```python
from build123d import *

# Parameters (mm, degrees)
F0_R     = 177.8
F1_DEPTH = 76.2
F2_R     = 88.9
F3_DEPTH = 254
F4_R     = 69.85
F5_DEPTH = 254
F6_W     = 462.104425
F6_H     = 46.355292
F6_W_2   = 466.450229
F6_H_2   = 34.23076
F7_DEPTH = 254
F8_R     = 158.592368
F9_DEPTH = 12.7


with BuildPart() as f1:
    # F0 (on Top) → F1 (new body)
    with BuildSketch(Plane.XY):
        Circle(F0_R)
    extrude(amount=F1_DEPTH)

    # F2 (on face) → F3 (cut)
    with BuildSketch(Plane.XY.offset(76.2)):
        Circle(F2_R)
    extrude(amount=-F3_DEPTH, mode=Mode.SUBTRACT)

    # F4 (on face) → F5 (cut)
    with BuildSketch(Plane.XY.offset(76.2)):
        with Locations((0, 177.8)):
            Circle(F4_R)
        with Locations((0, -177.8)):
            Circle(F4_R)
    extrude(amount=-F5_DEPTH, mode=Mode.SUBTRACT)

    # F6 (on face) → F7 (cut)
    with BuildSketch(Plane.XY.offset(76.2)):
        with Locations((-1.086809, 155.526124)):
            Rectangle(F6_W, F6_H)
        with Locations((1.086094, -146.964084)):
            Rectangle(F6_W_2, F6_H_2)
    extrude(amount=-F7_DEPTH, mode=Mode.SUBTRACT)

    # F8 (on face) → F9 (cut)
    with BuildSketch(Plane.XY.offset(76.2)):
        Circle(F8_R)
    extrude(amount=-F9_DEPTH, mode=Mode.SUBTRACT)


solid = f1.part
```
Input: part model. Units: mm. Frame: model coordinates. A direction names the side the tool comes from. Coordinates: 2 decimals unless noted, no trailing zeros. Write each loop counter-clockwise with the first axis right and the second up, starting at its lowest first coordinate (ties: lowest second). Pieces come first, ordered by that corner, then holes. Notation, with made-up numbers: (86, 88) - (138, 88) arc R24 ccw to (138, 106) - close; hole circle Ø10 at (-28, -26.5). An arc over 180 degrees is marked (long way). Put each result on its own line as item: value. Start each with the question number.
1) Mould query, pull axis X, two halves, no side actions, for faces 3 (the face through (-177.757, 3.914, 37.567)), 4 (the face through (-86, 132.348, 39)), 5 (the face through (0.796, -107.955, 32.194)). Classes: pulls with the +X half, pulls with the -X half, needs draft (parallel to the pull), parting line crosses it, or undercut.
2) Cut plane B-B (z = 27). Return the cut outline in (x, y).
3) Ray query, L1, parallel to Y at x = 0, z = 44; L2, parallel to Z at x = 75, y = 49.5; L3, parallel to Y at x = 61, z = 31.5. Return the intervals inside material, ascending.
4) Cut plane A-A (x = 0). Return the cut outline in (y, z).
5) Reachability of faces 1 (the face through (84.795, 26.703, 32.194)), 2 (the face through (-73, -55, 63.5)) from +Z, -Z, +X, -X, +Y, -Y: full face, straight path, thin tool, end or side. Return the list, or none.
6) Cut plane C-C (y = 0). Return the cut outline in (x, z), plus the area to 3 significant figures.
7) Cut plane D-D (y = -103). Return the cut outline in (x, z), plus the area to 3 significant figures.
8) Contact query for flat-ended pins moving along their axis: pin 1 (3 mm diameter, centred on x = -76.5, y = 73.5, fed in from +Z); pin 2 (5 mm diameter, centred on y = 99.5, z = 21.5, fed in from -X); pin 3 (5 mm diameter, centred on y = -77, z = 35.5, fed in from +X). Output: stop coordinate, or through.
Resolved:
1. face 3: pulls with the -X half
1. face 4: needs draft
1. face 5: undercut
2. outline: (-121.46, -129.85) - (-50.79, -129.85) arc R69.85 cw to (50.79, -129.85) - (121.46, -129.85) arc R177.8 ccw to (118.73, 132.35) - (53.04, 132.35) arc R69.85 cw to (-53.04, 132.35) - (-118.73, 132.35) arc R177.8 ccw to start; hole circle Ø177.8 at (0, 0)
3. L1: y = -107.95 to -88.9, 88.9 to 107.95
3. L2: z = 0 to 63.5
3. L3: y = -129.85 to -64.67, 64.67 to 132.35
4. outline: (-107.95, 0) - (-88.9, 0) - (-88.9, 63.5) - (-107.95, 63.5) - close; (88.9, 0) - (107.95, 0) - (107.95, 63.5) - (88.9, 63.5) - close
5. face 1: +Z, -Z
5. face 2: +Z
6. outline: (-177.8, 0) - (-88.9, 0) - (-88.9, 63.5) - (-158.59, 63.5) - (-158.59, 76.2) - (-177.8, 76.2) - close; (88.9, 0) - (177.8, 0) - (177.8, 76.2) - (158.59, 76.2) - (158.59, 63.5) - (88.9, 63.5) - close
6. area: 11,800 mm2
7. outline: (-144.93, 0) - (144.93, 0) - (144.93, 76.2) - (120.59, 76.2) - (120.59, 63.5) - (-120.59, 63.5) - (-120.59, 76.2) - (-144.93, 76.2) - close
7. area: 19,000 mm2
8. pin 1: stops at z = 63.5
8. pin 2: stops at x = -149.01
8. pin 3: stops at x = 161.44
